```python
from build123d import *

# Parameters (mm, degrees)
SKETCH1_W           = 20
SKETCH1_H           = 180
BOSS_EXTRUDE1_DEPTH = 30
SKETCH2_W           = 40
SKETCH2_H           = 40
BOSS_EXTRUDE2_DEPTH = 20
FILLET1_R           = 10


with BuildPart() as part:
    # Sketch1 → Boss-Extrude1 (new body)
    with BuildSketch(Plane.XY):
        with Locations((-20, -90)):
            Rectangle(SKETCH1_W, SKETCH1_H)
    extrude(amount=BOSS_EXTRUDE1_DEPTH)

    # Sketch2 → Boss-Extrude2 (add)
    with BuildSketch(Plane.XY):
        with Locations((-10, -160)):
            Rectangle(SKETCH2_W, SKETCH2_H)
    extrude(amount=-BOSS_EXTRUDE2_DEPTH)

    # Fillet1
    fillet1_edges = [part.edges().sort_by_distance(p)[0] for p in [
        (10, -140, -10),
        (-20, 0, 30),
    ]]
    fillet(fillet1_edges, radius=FILLET1_R)


solid = part.part
```
Could you check a few things on this model? Use its own coordinates, in mm. A direction names the side the tool comes from. Round coordinates to 2 decimals unless told otherwise and drop trailing zeros. Write each loop counter-clockwise with the first axis right and the second up, starting at its lowest first coordinate (ties: lowest second). Pieces come first, ordered by that corner, then holes.
(1) Suppose I cut it at A-A on z = -16. Write out the boundary of the cut face in (x, y), and give its area (3 significant figures).
Findings below:
outline: (-30, -180) - (10, -180) - (10, -150) arc R10 ccw to (0, -140) - (-30, -140) - close
area: 1,580 mm2
(2) Suppose I cut it at C-C on y = -155. Write out the boundary of the cut face in (x, z).
Findings below:
outline: (-30, -20) - (10, -20) - (10, 0) - (-10, 0) - (-10, 30) - (-30, 30) - close
(3) Suppose I cut it at B-B on x = -12.5. Write out the boundary of the cut face in (y, z).
Findings below:
outline: (-180, -20) - (-140, -20) - (-140, 0) - (0, 0) - (0, 20) arc R10 ccw to (-10, 30) - (-180, 30) - close
(4) Which directions (+Z, -Z, +X, -X, +Y, -Y) give clear straight access to the entire face, cutting with the end or side of a thin tool? Please do faces 1 (the face through (0, -160, 0)), 2 (the face through (-15, -140, -10)), 3 (the face through (-20, 0, 10)).
Findings below:
face 1: +Z, +X, +Y, -Y
face 2: -Z, +X, -X, +Y
face 3: +Z, -Z, +X, -X, +Y
(5) Suppose I cut it at D-D on x = -3. Write out the boundary of the cut face in (y, z), and give its area (3 significant figures).
Findings below:
outline: (-180, -20) - (-140, -20) - (-140, 0) - (-180, 0) - close
area: 800 mm2
(6) For pin 1 (10 mm diameter, centred on x = -21.5, z = -7.5, fed in from +Y); pin 2 (24 mm diameter, centred on y = -59, z = 8, fed in from +X); pin 3 (5 mm diameter, centred on x = -25, y = -95, fed in from -Z), each with a flat end and sliding along its axis, tell me the tip position at first contact or that it passes through.
Findings below:
pin 1: stops at y = -140
pin 2: stops at x = -10
pin 3: stops at z = 0
(7) If I drill on probe 1 along X at (y, z) = (-33.5, 28); probe 2 along Z at (x, y) = (-20.5, -38); probe 3 along Y at (x, z) = (-4, -0.5), over which ranges is the centre line in solid material (lowest first)?
Findings below:
probe 1: x = -30 to -10
probe 2: z = 0 to 30
probe 3: y = -180 to -140
